Geometry check sheet. Reference: the model listing, model coordinates, mm. Coordinates: 2 decimals unless noted, no trailing zeros. Loops run counter-clockwise (first coordinate to the right, second up) from the corner with the lowest first, then second, coordinate; pieces in that order, holes last. Notation, with made-up numbers: (-36.75, 16) -> (2.25, 16) arc R25 ccw to (2.25, 29) -> close; hole circle Ø10 at (-13.5, 62). An arc over 180 degrees is marked (long way). Answer as a JSON object with one key per item and string values.
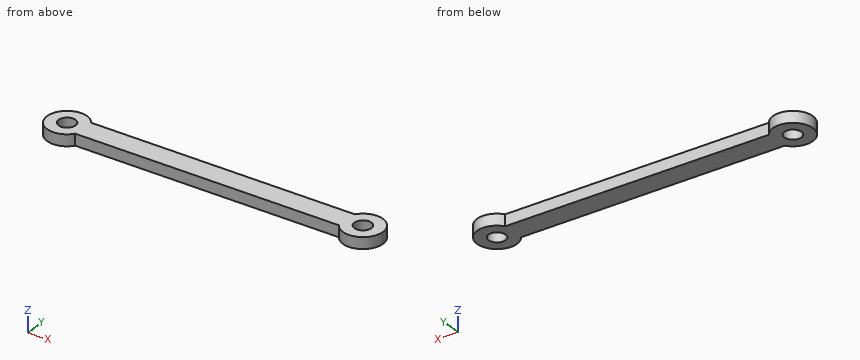
from build123d import *

# Parameters (mm, degrees)
CROQUIS1_R              = 1.5
SALIENTE_EXTRUIR1_DEPTH = 2


with BuildPart() as part:
    # Croquis1 → Saliente-Extruir1 (new body)
    with BuildSketch(Plane.XY):
        with BuildLine():
            ThreePointArc((-22.872281323, 0), (-23.032896303, -1.048097173), (-23.5, -2))
            Line((-23.5, -2), (23.5, -2))
            ThreePointArc((23.5, -2), (22.872281323, 0), (23.5, 2))
            Line((23.5, 2), (-23.5, 2))
            ThreePointArc((-23.5, 2), (-23.032896303, 1.048097173), (-22.872281323, 0))
        make_face()
        with BuildLine():
            ThreePointArc((-23.5, 2), (-29.872281323, 0), (-23.5, -2))
            Line((-23.5, -2), (-23.5, 2))
        make_face()
        with Locations((-26.372281323, 0)):
            Circle(CROQUIS1_R, mode=Mode.SUBTRACT)
        with BuildLine():
            Line((23.5, 2), (23.5, -2))
            ThreePointArc((23.5, -2), (27.420378496, -3.339385021), (29.872281323, 0))
            ThreePointArc((29.872281323, 0), (27.420378496, 3.339385021), (23.5, 2))
        make_face()
        with Locations((26.372281323, 0)):
            Circle(CROQUIS1_R, mode=Mode.SUBTRACT)
        with BuildLine():
            Line((-23.5, 2), (-23.5, -2))
            ThreePointArc((-23.5, -2), (-23.032896303, -1.048097173), (-22.872281323, 0))
            ThreePointArc((-22.872281323, 0), (-23.032896303, 1.048097173), (-23.5, 2))
        make_face()
        with BuildLine():
            ThreePointArc((23.5, 2), (22.872281323, 0), (23.5, -2))
            Line((23.5, -2), (23.5, 2))
        make_face()
    extrude(amount=SALIENTE_EXTRUIR1_DEPTH)


solid = part.part
1. Thickness scan on probe 1 along X at (y, z) = (-0.5, 0.8); probe 2 along Y at (x, z) = (1, 0.6); probe 3 along Y at (x, z) = (27, 0.1). Record the ranges inside material, lowest first. Write a range as from..to.
Evaluation:
{"probe 1": "x = -29.84..-27.79, -24.96..24.96, 27.79..29.84", "probe 2": "y = -2..2", "probe 3": "y = -3.44..-1.36, 1.36..3.44"}
2. Section check D-D, the plane x = -3. Record the boundary of the cut face in (y, z).
Evaluation:
{"outline": "(-2, 0) -> (2, 0) -> (2, 2) -> (-2, 2) -> close"}
3. Section check A-A, the plane z = 1.35. Record the boundary of the cut face in (x, y).
Evaluation:
{"outline": "(-23.5, -2) -> (23.5, -2) arc R3.5 ccw (long way) to (23.5, 2) -> (-23.5, 2) arc R3.5 ccw (long way) to start; hole circle Ø3 at (-26.37, 0); hole circle Ø3 at (26.37, 0)"}
4. Section check C-C, the plane y = -0.5. Record the boundary of the cut face in (x, z), then the cut area to 3 significant figures.
Evaluation:
{"outline": "(-29.84, 0) -> (-27.79, 0) -> (-27.79, 2) -> (-29.84, 2) -> close; (-24.96, 0) -> (24.96, 0) -> (24.96, 2) -> (-24.96, 2) -> close; (27.79, 0) -> (29.84, 0) -> (29.84, 2) -> (27.79, 2) -> close", "area": "108 mm^2"}
5. Section check B-B, the plane y = 3. Record the boundary of the cut face in (x, z), then the cut area to 3 significant figures.
Evaluation:
{"outline": "(-28.18, 0) -> (-24.57, 0) -> (-24.57, 2) -> (-28.18, 2) -> close; (24.57, 0) -> (28.18, 0) -> (28.18, 2) -> (24.57, 2) -> close", "area": "14.4 mm^2"}
6. Depth check by flat-ended pin: P1, Ø1.8, axis at x = -26.37, y = 0, coming from the -Z side; P2, Ø0.6, axis at x = -10, z = 1.5, coming from the -Y side. Enter the tip coordinate at first touch or a pass-through.
Evaluation:
{"P1": "passes through", "P2": "stops at y = -2"}
